Geometry check sheet. Reference: the model listing, model coordinates, mm. A direction names the side the tool comes from. Coordinates: 2 decimals unless noted, no trailing zeros. Loops run counter-clockwise (first coordinate to the right, second up) from the corner with the lowest first, then second, coordinate; pieces in that order, holes last. Notation, with made-up numbers: (13.5, -3) -> (67.5, -3) arc R13 cw to (67.5, 3) -> close; hole circle Ø4 at (80.5, 13). An arc over 180 degrees is marked (long way). Answer as a JSON object with one key per item and string values.
from build123d import *

# Parameters (mm, degrees)
SKETCH1_R                = 13.97
SKETCH1_R_2              = 1.275
BOSS_EXTRUDE1_DEPTH      = 3.048
BOSS_EXTRUDE2_DEPTH      = 46.99
BOSS_EXTRUDE2_DEPTH_BACK = 3.048
SKETCH2_R                = 7.874
SKETCH2_R_2              = 1.275
CUT_EXTRUDE2_DEPTH       = 117.959760362
SKETCH6_R                = 8.89
SKETCH6_R_2              = 4.191
BOSS_EXTRUDE3_DEPTH      = 4.572
FILLET2_R                = 3.048
SKETCH7_W                = 199.707818202
SKETCH7_H                = 58.861251681
CUT_EXTRUDE3_DEPTH       = 117.959760362


with BuildPart() as part:
    # Sketch1 → Boss-Extrude1 (new body)
    with BuildSketch(Plane(origin=(0, 0, 0), x_dir=(1, 0, 0), z_dir=(0, 1, 0))):
        with Locations(Location((0, 0, 0), (0, 0, 90))):
            Circle(SKETCH1_R)
        with Locations(Location((0, 9.5, 0), (0, 0, 90))):
            Circle(SKETCH1_R_2, mode=Mode.SUBTRACT)
        with Locations(Location((9.5, 0, 0), (0, 0, 90))):
            Circle(SKETCH1_R_2, mode=Mode.SUBTRACT)
        with Locations(Location((0, -9.5, 0), (0, 0, 90))):
            Circle(SKETCH1_R_2, mode=Mode.SUBTRACT)
        with Locations(Location((-9.5, 0, 0), (0, 0, 90))):
            Circle(SKETCH1_R_2, mode=Mode.SUBTRACT)
    extrude(amount=BOSS_EXTRUDE1_DEPTH)

    # Sketch2 → Boss-Extrude2 (add, two sides: drawn at the far end of the back side and taken through both)
    with BuildSketch(Plane(origin=(0, 3.048, 0), x_dir=(1, 0, 0), z_dir=(0, 1, 0)).offset(-BOSS_EXTRUDE2_DEPTH_BACK)):
        with BuildLine():
            Line((-96.52, -14.605), (96.52, -14.605))
            ThreePointArc((96.52, -14.605), (100.112102448, -13.117102448), (101.6, -9.525))
            Line((101.6, -9.525), (101.6, 9.525))
            ThreePointArc((101.6, 9.525), (100.112102448, 13.117102448), (96.52, 14.605))
            Line((96.52, 14.605), (-96.52, 14.605))
            ThreePointArc((-96.52, 14.605), (-100.112102448, 13.117102448), (-101.6, 9.525))
            Line((-101.6, 9.525), (-101.6, -9.525))
            ThreePointArc((-101.6, -9.525), (-100.112102448, -13.117102448), (-96.52, -14.605))
        make_face()
        with Locations(Location((-88.9, 0, 0), (0, 0, 270))):
            Circle(SKETCH2_R, mode=Mode.SUBTRACT)
        with Locations(Location((88.9, 0, 0), (0, 0, 270))):
            Circle(SKETCH2_R, mode=Mode.SUBTRACT)
        with Locations(Location((9.5, 0, 0), (0, 0, 90))):
            Circle(SKETCH2_R_2, mode=Mode.SUBTRACT)
        with Locations(Location((0, 9.5, 0), (0, 0, 90))):
            Circle(SKETCH2_R_2, mode=Mode.SUBTRACT)
        with Locations(Location((-9.5, 0, 0), (0, 0, 90))):
            Circle(SKETCH2_R_2, mode=Mode.SUBTRACT)
        with Locations(Location((0, -9.5, 0), (0, 0, 90))):
            Circle(SKETCH2_R_2, mode=Mode.SUBTRACT)
    extrude(amount=BOSS_EXTRUDE2_DEPTH + BOSS_EXTRUDE2_DEPTH_BACK)

    # Sketch5 → Cut-Extrude2 (cut, through all)
    with BuildSketch(Plane(origin=(0, 0, -14.605), x_dir=(-1, 0, 0), z_dir=(0, 0, -1))):
        Polygon((-76.2, 5.08), (0, 5.08), (76.2, 5.08), (76.2, 50.038), (-76.2, 50.038), align=None)
    extrude(amount=-CUT_EXTRUDE2_DEPTH, mode=Mode.SUBTRACT)

    # Sketch6 → Boss-Extrude3 (add)
    # profile 1 of 2: a face of its own
    with BuildSketch(Plane.XZ):
        with Locations((-88.9, 0)):
            Circle(SKETCH6_R)
        with Locations(Location((-88.9, 0, 0), (0, 0, 270))):
            Circle(SKETCH6_R_2, mode=Mode.SUBTRACT)
    # profile 2 of 2: a face of its own
    with BuildSketch(Plane.XZ):
        with Locations((88.9, 0)):
            Circle(SKETCH6_R)
        with Locations(Location((88.9, 0, 0), (0, 0, 270))):
            Circle(SKETCH6_R_2, mode=Mode.SUBTRACT)
    extrude(amount=-BOSS_EXTRUDE3_DEPTH)

    # Fillet2
    fillet2_edges = [part.edges().sort_by_distance(p)[0] for p in [
        (-76.2, 5.08, 0),
        (76.2, 5.08, 0),
    ]]
    fillet(fillet2_edges, radius=FILLET2_R)

    # Sketch7 → Cut-Extrude3 (cut, through all)
    with BuildSketch(Plane(origin=(0, 0, -14.605), x_dir=(-1, 0, 0), z_dir=(0, 0, -1))):
        with Locations((30.0995037, 26.703530829)):
            Rectangle(SKETCH7_W, SKETCH7_H)
    extrude(amount=-CUT_EXTRUDE3_DEPTH, mode=Mode.SUBTRACT)


solid = part.part
1. Section check B-B, the plane z = 0. Record the boundary of the cut face in (x, y).
Evaluation:
{"outline": "(69.75, 0) -> (84.71, 0) -> (84.71, 4.57) -> (81.03, 4.57) -> (81.03, 50.04) -> (76.2, 50.04) -> (76.2, 8.13) arc R3.05 cw to (73.15, 5.08) -> (69.75, 5.08) -> close; (93.09, 0) -> (101.6, 0) -> (101.6, 50.04) -> (96.77, 50.04) -> (96.77, 4.57) -> (93.09, 4.57) -> close"}
2. Tool access check on faces 4 (the face through (84.81, 2.25, 0.91)), 5 (the face through (76.2, 29, 0)), 6 (the face through (92.3, 4.572, -3.4)). Record the directions out of +Z, -Z, +X, -X, +Y, -Y that give a thin tool (end or side, any length) a straight path to the whole face; none if there is none.
Evaluation:
{"face 4": "+Y, -Y", "face 5": "+Z, -Z, -X, +Y", "face 6": "+Y"}
3. Thickness scan on probe 1 along Z at (x, y) = (88.9, 17) (3 decimals); probe 2 along X at (y, z) = (22, 0); probe 3 along Y at (x, z) = (88, -6.75). Record the ranges inside material, lowest first. Write a range as from..to.
Evaluation:
{"probe 1": "z = -14.605..-7.874, 7.874..14.605", "probe 2": "x = 76.2..81.03, 96.77..101.6", "probe 3": "y = 0..4.57"}
4. Depth check by flat-ended pin: P1, Ø4, axis at y = 22, z = 5, coming from the -X side; P2, Ø1, axis at x = 85.5, z = 4, coming from the +Y side; P3, Ø10, axis at x = 86, z = 0.5, coming from the +Y side; P4, Ø5, axis at x = 88.9, z = 0, coming from the +Y side. Enter the tip coordinate at first touch or a pass-through.
Evaluation:
{"P1": "stops at x = 76.2", "P2": "stops at y = 4.57", "P3": "stops at y = 50.04", "P4": "passes through"}
5. Section check C-C, the plane y = 9. Record the boundary of the cut face in (x, z) (3 decimals), then the cut area to 3 significant figures.
Evaluation:
{"outline": "(76.2, -14.605) -> (96.52, -14.605) arc R5.08 ccw to (101.6, -9.525) -> (101.6, 9.525) arc R5.08 ccw to (96.52, 14.605) -> (76.2, 14.605) -> close; hole circle Ø15.748 at (88.9, 0)", "area": "536 mm^2"}
6. Mould release check, pull along Z, two halves, no side actions. Record for faces 1 (the face through (86, 25, -14.605)), 2 (the face through (81.213, 26.987, -1.707)), 3 (the face through (85, 0, -3)): released by +Z, released by -Z, zero draft, split by the parting line, or undercut.
Evaluation:
{"face 1": "released by -Z", "face 2": "undercut", "face 3": "zero draft"}
7. Section check D-D, the plane z = -5.25. Record the boundary of the cut face in (x, y).
Evaluation:
{"outline": "(69.75, 0) -> (101.6, 0) -> (101.6, 50.04) -> (94.77, 50.04) -> (94.77, 4.57) -> (83.03, 4.57) -> (83.03, 50.04) -> (76.2, 50.04) -> (76.2, 8.13) arc R3.05 cw to (73.15, 5.08) -> (69.75, 5.08) -> close"}
8. Section check A-A, the plane x = 88.9. Record the boundary of the cut face in (y, z) (3 decimals).
Evaluation:
{"outline": "(0, -14.605) -> (50.038, -14.605) -> (50.038, -7.874) -> (4.572, -7.874) -> (4.572, -4.191) -> (0, -4.191) -> close; (0, 4.191) -> (4.572, 4.191) -> (4.572, 7.874) -> (50.038, 7.874) -> (50.038, 14.605) -> (0, 14.605) -> close"}
